Geometry: final body of the model. Coordinates: model frame, mm. A direction names the side the tool comes from. Coordinates: 2 decimals unless noted, no trailing zeros. Order: outer loops, then holes, each group sorted by start corner. A loop starts at its lowest first (then second) coordinate and runs counter-clockwise, first axis right, second up. Notation, with made-up numbers: M -25,-31.5 L 14,-31.5 A22 ccw 14,-4.5 Z; hole C -26,15 d6. An arc over 180 degrees is marked long. One line per question, with ' | ' between items.
from build123d import *

# Parameters (mm, degrees)
F1_DEPTH = 30


with BuildPart() as f1:
    # F0 (on Front) → F1 (new body)
    with BuildSketch(Plane.XZ):
        with BuildLine():
            ThreePointArc((-35.692446, -10.797127), (-41.286589, -35.884078), (-17.804858, -46.336725))
            Line((-17.804858, -46.336725), (32.195142, -46.336725))
            ThreePointArc((32.195142, -46.336725), (51.423961, -32.524361), (44.473924, -9.891954))
            ThreePointArc((44.473924, -9.891954), (44.025197, -9.560505), (43.567529, -9.241517))
            ThreePointArc((43.567529, -9.241517), (32.195142, -5.755051), (20.822756, -9.241517))
            Line((20.822756, -9.241517), (15.829317, -9.49759))
            Line((15.829317, -9.49759), (16.125229, -15.267867))
            ThreePointArc((16.125229, -15.267867), (4.796341, -25.139633), (-7.482951, -16.478543))
            Line((-7.482951, -16.478543), (-7.482951, -9.49759))
            Line((-7.482951, -9.49759), (-12.482951, -9.49759))
            ThreePointArc((-12.482951, -9.49759), (-23.157559, -6.463665), (-33.832168, -9.49759))
            ThreePointArc((-33.832168, -9.49759), (-34.780484, -10.121339), (-35.692446, -10.797127))
        make_face()
        with BuildLine():
            Line((-35.692446, -9.49759), (-35.692446, -10.797127))
            ThreePointArc((-35.692446, -10.797127), (-34.780484, -10.121339), (-33.832168, -9.49759))
            Line((-33.832168, -9.49759), (-35.692446, -9.49759))
        make_face()
        with BuildLine():
            ThreePointArc((43.567529, -9.241517), (44.025197, -9.560505), (44.473924, -9.891954))
            Line((44.473924, -9.891954), (44.473924, -9.241517))
            Line((44.473924, -9.241517), (43.567529, -9.241517))
        make_face()
    extrude(amount=F1_DEPTH)


solid = f1.part
1. Section A-A, the plane z = -20. Output: boundary loops of the cut face in (x, y).
Response values:
outline: M -42.29,-30 L -5.77,-30 L -5.77,0 L -42.29,0 Z; M 14.12,-30 L 51.56,-30 L 51.56,0 L 14.12,0 Z
2. Section C-C, the plane x = -9. Output: boundary loops of the cut face in (y, z), and give its area (3 significant figures).
Response values:
outline: M -30,-46.34 L 0,-46.34 L 0,-9.5 L -30,-9.5 Z | area: 1,110 mm^2
3. Material intervals for line 1 (X direction, y = -1.5, z = -12.5); line 2 (X direction, y = -26.75, z = -18); line 3 (Z direction, x = -14.5, y = -22.25), sorted ascending. Write a range as [from, to].
Response values:
line 1: x = [-37.6, -7.48], [15.98, 47.3] | line 2: x = [-41.47, -6.91], [15.26, 50.82] | line 3: z = [-46.34, -8.4]
4. Pin query (flat end, axial travel): P1, Ø1, axis at y = -7, z = -21.5, coming from the +X side; P2, Ø4, axis at y = -4, z = -41, coming from the -X side; P3, Ø0.9, axis at x = -34.5, y = -14.5, coming from the +Z side. Return the tip coordinate at first contact, or that it passes through.
Response values:
P1: stops at x = 52.08 | P2: stops at x = -39.35 | P3: stops at z = -9.5
5. Access query for faces 4 (the face through (4, -30, -26)), 5 (the face through (18.361, -14.79, -9.368)), 6 (the face through (7, -15, -46.337)). Directions: +Z, -Z, +X, -X, +Y, -Y. A direction counts if a zero-diameter tool reaches every point of the face in a straight line with its end or side. Return the directions, or none.
Response values:
face 4: +Z, -Z, +X, -X, -Y | face 5: +Z, +Y, -Y | face 6: -Z, +X, +Y, -Y
6. Section B-B, the plane y = -23.75. Output: boundary loops of the cut face in (x, z).
Response values:
outline: M -35.69,-10.8 A20.3 ccw -17.8,-46.34 L 32.2,-46.34 A20.29 ccw 44.47,-9.89 L 44.47,-9.24 L 43.57,-9.24 A20.29 ccw 20.82,-9.24 L 15.83,-9.5 L 16.13,-15.27 A12.17 cw -7.48,-16.48 L -7.48,-9.5 L -12.48,-9.5 A20.3 ccw -33.83,-9.5 L -35.69,-9.5 Z
7. Draft query along Z for faces 1 (the face through (51.308, -14.79, -32.859)), 2 (the face through (15.975, -14.79, -12.342)), 3 (the face through (-35, -15, -9.498)). Return one class per face: pulls with the +Z half, pulls with the -Z half, needs draft (parallel to the pull), parting line crosses it, or undercut.
Response values:
face 1: parting line crosses it | face 2: undercut | face 3: pulls with the +Z half
8. Section D-D, the plane z = -12. Output: boundary loops of the cut face in (x, y), and give its area (3 significant figures).
Response values:
outline: M -37.09,-30 L -7.48,-30 L -7.48,0 L -37.09,0 Z; M 15.96,-30 L 46.84,-30 L 46.84,0 L 15.96,0 Z | area: 1,810 mm^2
